```python
from build123d import *

# Parameters (mm, degrees)
F_4_BAR_LINKAGE_NON_DRIVEN_BAR_OUTLINE_R   = 3.3655
F_4_BAR_LINKAGE_NON_DRIVEN_BAR_OUTLINE_R_2 = 0.877000024
F_4_BAR_LINKAGE_NON_DRIVEN_BAR_DEPTH       = 9.525
BOSS_EXTRUDE2_DEPTH                        = 9.525
CUT_EXTRUDE1_DEPTH                         = 91.807220253
FILLET1_R                                  = 3.175
FILLET3_R                                  = 3.175


# Read off the part's stored shape, not the designer's step: 4 bar linkage non-driven bar
with BuildPart() as part:
    # 4 bar linkage non-driven bar outline → 4 bar linkage non-driven bar (new body)
    with BuildSketch(Plane.XY):
        with BuildLine():
            ThreePointArc((-6.35, 0), (0, -6.35), (6.35, 0))
            Line((6.35, 0), (6.35, 82.55))
            ThreePointArc((6.35, 82.55), (0, 88.9), (-6.35, 82.55))
            Line((-6.35, 82.55), (-6.35, 0))
        make_face()
        Circle(F_4_BAR_LINKAGE_NON_DRIVEN_BAR_OUTLINE_R, mode=Mode.SUBTRACT)
        with Locations((0, 6.99999997)):
            Circle(F_4_BAR_LINKAGE_NON_DRIVEN_BAR_OUTLINE_R_2, mode=Mode.SUBTRACT)
        with Locations((0, 16.000000004)):
            Circle(F_4_BAR_LINKAGE_NON_DRIVEN_BAR_OUTLINE_R_2, mode=Mode.SUBTRACT)
        with Locations((0, 82.55)):
            Circle(F_4_BAR_LINKAGE_NON_DRIVEN_BAR_OUTLINE_R, mode=Mode.SUBTRACT)
    extrude(amount=F_4_BAR_LINKAGE_NON_DRIVEN_BAR_DEPTH)

    # Sketch2 → Boss-Extrude2 (add)
    with BuildSketch(Plane.XY.offset(9.525)):
        with BuildLine():
            Line((6.35, 17.200322169), (6.35, 46.299677831))
            ThreePointArc((6.35, 46.299677831), (15.875, 31.75), (6.35, 17.200322169))
        make_face()
    extrude(amount=-BOSS_EXTRUDE2_DEPTH)

    # Sketch1 → Cut-Extrude1 (cut, through all)
    with BuildSketch(Plane.XY.offset(9.525)):
        with BuildLine():
            Line((-0.096808673, 39.9415), (-6.35, 39.9415))
            Line((-6.35, 39.9415), (-6.35, 23.5585))
            Line((-6.35, 23.5585), (-0.096808673, 23.5585))
            ThreePointArc((-0.096808673, 23.5585), (8.094691327, 31.75), (-0.096808673, 39.9415))
        make_face()
    extrude(amount=-CUT_EXTRUDE1_DEPTH, mode=Mode.SUBTRACT)

    # Fillet1
    fillet1_edges = [part.edges().sort_by_distance(p)[0] for p in [
        (-6.35, 23.5585, 4.7625),
        (-6.35, 39.9415, 4.7625),
    ]]
    fillet(fillet1_edges, radius=FILLET1_R)

    # Fillet3
    fillet3_edges = [part.edges().sort_by_distance(p)[0] for p in [
        (6.35, 46.299677831, 4.7625),
        (6.35, 17.200322169, 4.7625),
    ]]
    fillet(fillet3_edges, radius=FILLET3_R)


solid = part.part
```
The model under review builds one solid part; all positions refer to its coordinate system, in mm. A direction names the side the tool comes from. Coordinates: 2 decimals unless noted, no trailing zeros. Write each loop counter-clockwise with the first axis right and the second up, starting at its lowest first coordinate (ties: lowest second). Pieces come first, ordered by that corner, then holes.
1) We need section A-A on z = 8.25. Count the separate pieces of the cut face and the enclosed holes in it, then the cut area to 3 significant figures.
2) We need section D-D on x = 10.75. State the section outline as (y, z) points (3 decimals).
3) We need section B-B on x = 4.5. State the section outline as (y, z) points (3 decimals), then the cut area to 3 significant figures.
4) To check wall thickness, follow probe 1 along Y at (x, z) = (0, 2); probe 2 along Y at (x, z) = (-1, 2.5); probe 3 along Y at (x, z) = (1.75, 3.25). State the ranges of each line that lie inside material, in increasing order.
5) Machinability: for faces 4 (the face through (-5.4, 40.85, 4.7)), 5 (the face through (-0.19, 6.144, 4.696)), 6 (the face through (6.35, 65, 5)), which of the approach directions +Z, -Z, +X, -X, +Y, -Y give a long, thin tool a straight path to every point of the face, cutting with its end or side? Answer none if there is none.
6) We need section C-C on y = 31.75. State the section outline as (x, z) points (3 decimals), then the cut area to 3 significant figures.
7) The part is to be moulded in two halves that separate along Y. For faces 1 (the face through (-0.438, 85.887, 4.696)), 2 (the face through (-6.35, 63, 5)), 3 (the face through (6.787, 46.64, 4.696)), say which applies: pulls with the +Y half, pulls with the -Y half, needs draft (parallel to the pull), parting line crosses it, or undercut.
8) Clearance check with flat-ended pins moving along their axes: pin 1 Ø3 at (y, z) = (54, 5.5) entering from +X; pin 2 Ø5 at (x, y) = (3.5, 60) entering from -Z; pin 3 Ø2 at (x, z) = (5.5, 2.5) entering from +Y; pin 4 Ø1.5 at (x, z) = (-2, 2.5) entering from -Y. State where each tip first meets the part, or that it passes through.
Answer list:
1. separate pieces: 1
1. enclosed holes: 4
1. area: 1,090 mm2
2. outline: (20.069, 0) - (43.431, 0) - (43.431, 9.525) - (20.069, 9.525) - close
3. outline: (-4.48, 0) - (24.97, 0) - (24.97, 9.525) - (-4.48, 9.525) - close; (38.53, 0) - (87.03, 0) - (87.03, 9.525) - (38.53, 9.525) - close
3. area: 742 mm2
4. probe 1: y = -6.35 to -3.37, 3.37 to 6.12, 7.88 to 15.12, 16.88 to 23.56, 39.94 to 79.18, 85.92 to 88.9
4. probe 2: y = -6.27 to -3.21, 3.21 to 23.56, 39.94 to 79.34, 85.76 to 88.82
4. probe 3: y = -6.1 to -2.87, 2.87 to 23.77, 39.73 to 79.68, 85.42 to 88.65
5. face 4: +Z, -Z, -X
5. face 5: +Z, -Z
5. face 6: +Z, -Z, +X, +Y
6. outline: (8.095, 0) - (15.875, 0) - (15.875, 9.525) - (8.095, 9.525) - close
6. area: 74.1 mm2
7. face 1: undercut
7. face 2: needs draft
7. face 3: pulls with the +Y half
8. pin 1: stops at x = 6.35
8. pin 2: stops at z = 0
8. pin 3: stops at y = 87.03
8. pin 4: stops at y = -6.23
